Autodesk Inventor part; units mm, degrees
ref_plane "YZ Plane" through (0, 0, 0) normal (1, 0, 0) x (0, 1, 0)
ref_plane "XZ Plane" through (0, 0, 0) normal (0, 1, 0) x (-1, 0, 0)
ref_plane "XY Plane" through (0, 0, 0) normal (0, 0, 1) x (1, 0, 0)
sketch "Esquisse1" plane through (0, 0, 0) normal (0, 1, 0) x (-1, 0, 0)
  line L0 (0, 0) -> (12, 0)
  line L1 (12, 0) -> (12, -10)
  line L2 (12, -10) -> (0, -10)
  line L3 (0, -10) -> (0, 0)
  dimension "d0" = 10
  dimension "d1" = 12
extrude "Extrusion1" add sketch "Esquisse1" along normal blind 25.6
sketch "Esquisse2" plane through (0, 25.6, 0) normal (0, 1, 0) x (1, 0, 0)
  line L0 (-12, 0) -> (0, 0) construction
  line L1 (0, 0) -> (0, 10) construction
  line L2 (0, 10) -> (-12, 10) construction
  line L3 (-12, 10) -> (-12, 0) construction
  line L4 (-12, 5) -> (0, 5) construction
  line L5 (0, 0) -> (0, 10) construction
  circle A0 centre (-6, 5) radius 1.5
  dimension "d4" = 3
extrude "Extrusion2" add sketch "Esquisse2" along normal blind 9
properties part number "motor"
Input: part model. Units: mm. Frame: model coordinates. A direction names the side the tool comes from. Coordinates: 2 decimals unless noted, no trailing zeros. Order: outer loops, then holes, each group sorted by start corner. A loop starts at its lowest first (then second) coordinate and runs counter-clockwise, first axis right, second up. Notation, with made-up numbers: M 75,48 L 114,48 A28 ccw 114,68 Z; hole C 42,37 d10. An arc over 180 degrees is marked long. Answer in a Markdown table with one row per item.
(1) Section query C-C, the plane x = -0.75. Output: boundary loops of the cut face in (y, z).
Numbers:
| item | result |
|---|---|
| outline | M 0,-10 L 25.6,-10 L 25.6,0 L 0,0 Z |
(2) Section query B-B, the plane z = -5. Output: boundary loops of the cut face in (x, y), plus the area to 3 significant figures.
Numbers:
| item | result |
|---|---|
| outline | M -12,0 L 0,0 L 0,25.6 L -4.5,25.6 L -4.5,34.6 L -7.5,34.6 L -7.5,25.6 L -12,25.6 Z |
| area | 334 mm^2 |
(3) Material intervals for line 1 (Y direction, x = -1.5, z = -7.5); line 2 (X direction, y = 29, z = -4.75), sorted ascending. Write a range as [from, to].
Numbers:
| item | result |
|---|---|
| line 1 | y = [0, 25.6] |
| line 2 | x = [-7.48, -4.52] |
(4) Contact query for a flat-ended pin moving along its axis: pin 1 Ø4 at (x, z) = (-1.5, -3) entering from +Y. Output: stop coordinate, or through.
Numbers:
| item | result |
|---|---|
| pin 1 | stops at y = 25.6 |
(5) Access query for faces 1 (the flat face through (-6, 13, 0)), 2 (the flat face through (-4.6, 25.6, -3.8)). Directions: +Z, -Z, +X, -X, +Y, -Y. A direction counts if a zero-diameter tool reaches every point of the face in a straight line with its end or side. Return the directions, or none.
Numbers:
| item | result |
|---|---|
| face 1 | +Z, +X, -X, +Y, -Y |
| face 2 | +Y |
(6) Section query A-A, the plane x = -6. Output: boundary loops of the cut face in (y, z).
Numbers:
| item | result |
|---|---|
| outline | M 0,-10 L 25.6,-10 L 25.6,-6.5 L 34.6,-6.5 L 34.6,-3.5 L 25.6,-3.5 L 25.6,0 L 0,0 Z |
